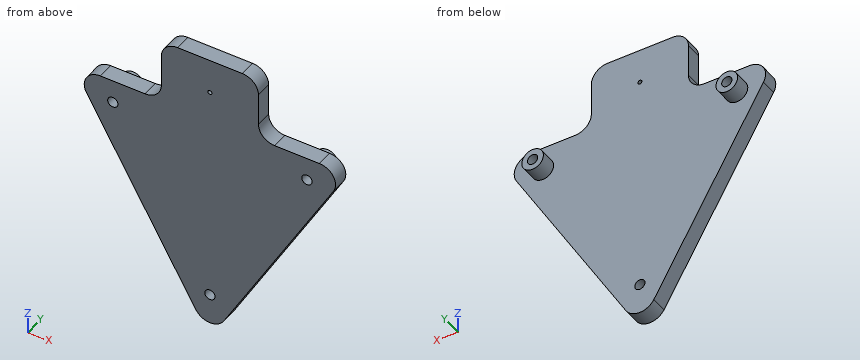
from build123d import *

# Parameters (mm, degrees)
SKETCH1_R           = 3.175
SKETCH1_R_2         = 1.25
BOSS_EXTRUDE2_DEPTH = 10
SKETCH2_R           = 6.675
SKETCH2_R_2         = 3.175
BOSS_EXTRUDE3_DEPTH = 10


with BuildPart() as part:
    # Sketch1 → Boss-Extrude2 (new body)
    with BuildSketch(Plane(origin=(0, 0, 0), x_dir=(1, 0, 0), z_dir=(0, 1, 0))):
        with BuildLine():
            Line((-67.679491924, 0), (-40, 0))
            ThreePointArc((-40, 0), (-32.928932188, -2.928932188), (-30, -10))
            Line((-30, -10), (-30, -30))
            ThreePointArc((-30, -30), (-27.071067812, -37.071067812), (-20, -40))
            Line((-20, -40), (20, -40))
            ThreePointArc((20, -40), (27.071067812, -37.071067812), (30, -30))
            Line((30, -30), (30, -10))
            ThreePointArc((30, -10), (32.928932188, -2.928932188), (40, 0))
            Line((40, 0), (67.679491924, 0))
            ThreePointArc((67.679491924, 0), (76.339745962, 5), (76.339745962, 15))
            Line((76.339745962, 15), (8.660254038, 132.224318643))
            ThreePointArc((8.660254038, 132.224318643), (0, 137.224318643), (-8.660254038, 132.224318643))
            Line((-8.660254038, 132.224318643), (-76.339745962, 15))
            ThreePointArc((-76.339745962, 15), (-76.339745962, 5), (-67.679491924, 0))
        make_face()
        with Locations(Location((-60, 14.43375673, 0), (0, 0, 270))):
            Circle(SKETCH1_R, mode=Mode.SUBTRACT)
        with Locations(Location((0, 118.356805184, 0), (0, 0, 270))):
            Circle(SKETCH1_R, mode=Mode.SUBTRACT)
        with Locations(Location((60, 14.43375673, 0), (0, 0, 270))):
            Circle(SKETCH1_R, mode=Mode.SUBTRACT)
        with Locations(Location((0, -18.450194816, 0), (0, 0, 270))):
            Circle(SKETCH1_R_2, mode=Mode.SUBTRACT)
    extrude(amount=BOSS_EXTRUDE2_DEPTH)

    # Sketch2 → Boss-Extrude3 (add)
    # profile 1 of 2: a face of its own
    with BuildSketch(Plane(origin=(0, 10, 0), x_dir=(1, 0, 0), z_dir=(0, 1, 0))):
        with Locations(Location((-60, 14.43375673, 0), (0, 0, 270))):
            Circle(SKETCH2_R)
        with Locations(Location((-60, 14.43375673, 0), (0, 0, 270))):
            Circle(SKETCH2_R_2, mode=Mode.SUBTRACT)
    # profile 2 of 2: a face of its own
    with BuildSketch(Plane(origin=(0, 10, 0), x_dir=(1, 0, 0), z_dir=(0, 1, 0))):
        with Locations(Location((60, 14.43375673, 0), (0, 0, 270))):
            Circle(SKETCH2_R)
        with Locations(Location((60, 14.43375673, 0), (0, 0, 270))):
            Circle(SKETCH2_R_2, mode=Mode.SUBTRACT)
    extrude(amount=BOSS_EXTRUDE3_DEPTH)


solid = part.part
CAD build for the part. Positions are in the model's coordinates, mm. Coordinates: 2 decimals unless noted, no trailing zeros. Loops run counter-clockwise (first coordinate to the right, second up) from the corner with the lowest first, then second, coordinate; pieces in that order, holes last. Notation, with made-up numbers: (-12, 45) - (37, 45) arc R24 cw to (37, 84) - close; hole circle Ø8 at (46, 84). An arc over 180 degrees is marked (long way). Use one line per item in the form item = value. Start each with the question number.
1) Band-saw the part on A-A (y = 7). State how many separate pieces and enclosed holes the cut face has, and give its area (3 significant figures).
2) Band-saw the part on D-D (z = -124.5). Give the cut face in (x, y).
3) Drill centre lines: L1, parallel to Y at x = -13.5, z = 19; L2, parallel to Z at x = 58.5, y = 18; L3, parallel to Z at x = 42, y = 9.5. Where is each one in solid material? Low to high. Write a range as from..to.
4) Flat gauge pins, fed straight in: pin 1 (5 mm diameter, centred on x = -60, z = -14.43, fed in from -Y); pin 2 (5 mm diameter, centred on y = 4, z = 19.5, fed in from +X); pin 3 (1.5 mm diameter, centred on x = 14.5, z = -30, fed in from +Y); pin 4 (3 mm diameter, centred on x = -52.5, y = 5.5, fed in from +Z). Where does each tip first touch, or does it go through?
5) Band-saw the part on C-C (x = 43.5). Give the cut face in (y, z), and give its area (3 significant figures).
6) Band-saw the part on B-B (x = -60). Give the cut face in (y, z), and give its area (3 significant figures).
Check values:
q1.separate_pieces = 1
q1.enclosed_holes = 4
q1.area = 14,600 mm2
q2.outline = (-13.12, 0) - (13.12, 0) - (13.12, 10) - (-13.12, 10) - close
q3.L1 = 0..10
q3.L2 = -20.94..-17.23, -11.64..-7.93
q3.L3 = -74.48..0
q4.pin_1 = through
q4.pin_2 = 30
q4.pin_3 = 10
q4.pin_4 = 0
q5.outline = (0, -71.88) - (10, -71.88) - (10, 0) - (0, 0) - close
q5.area = 719 mm2
q6.outline = (0, -43.3) - (10, -43.3) - (10, -21.11) - (20, -21.11) - (20, -17.61) - (0, -17.61) - close; (0, -11.26) - (20, -11.26) - (20, -7.76) - (10, -7.76) - (10, 0) - (0, 0) - close
q6.area = 440 mm2
